Answer from the drawing. Dimensions are ordinates in mm from the lowest x, y and z of the part. Coordinates: 2 decimals unless noted, no trailing zeros. Order: outer loops, then holes, each group sorted by start corner. A loop starts at its lowest first (then second) coordinate and runs counter-clockwise, first axis right, second up. Notation, with made-up numbers: (-7.5, -28) - (12.5, -28) arc R36 cw to (12.5, 6) - close; hole circle Ø8 at (-8, 65.25). An arc over 180 degrees is marked (long way). Use a Markdown table: item, result. Add a question column.
Item 1: The mould has two halves that part along X. Classify the marked faces 1, 2, 3 and 4: released by +X, released by -X, zero draft, split by the parting line, or undercut.
Item 2: The part is cut by section B-B, the plane y = 1.3. Give the vertices of the cut face in (x, z).
Item 3: Flat-ended cylindrical pins translate along their axes: P1, Ø1, axis at x = 3.5, z = 4, coming from the -Y side; P2, Ø3, axis at x = 7, z = 6, coming from the -Y side. Find the tip coordinate at first contact, or state that the pin passes through.
Item 4: Find the intervals of material crossed by line 1 along X through (y, z) = (2.8, 5); line 2 along Z through (x, y) = (5, 2.15) (1 decimal); line 3 along X through (y, z) = (1.8, 4.25) (1 decimal), in increasing order.
Item 5: The part is cut by section A-A, the plane z = 5. Give the vertices of the cut face in (x, y), then the cut area to 3 significant figures.
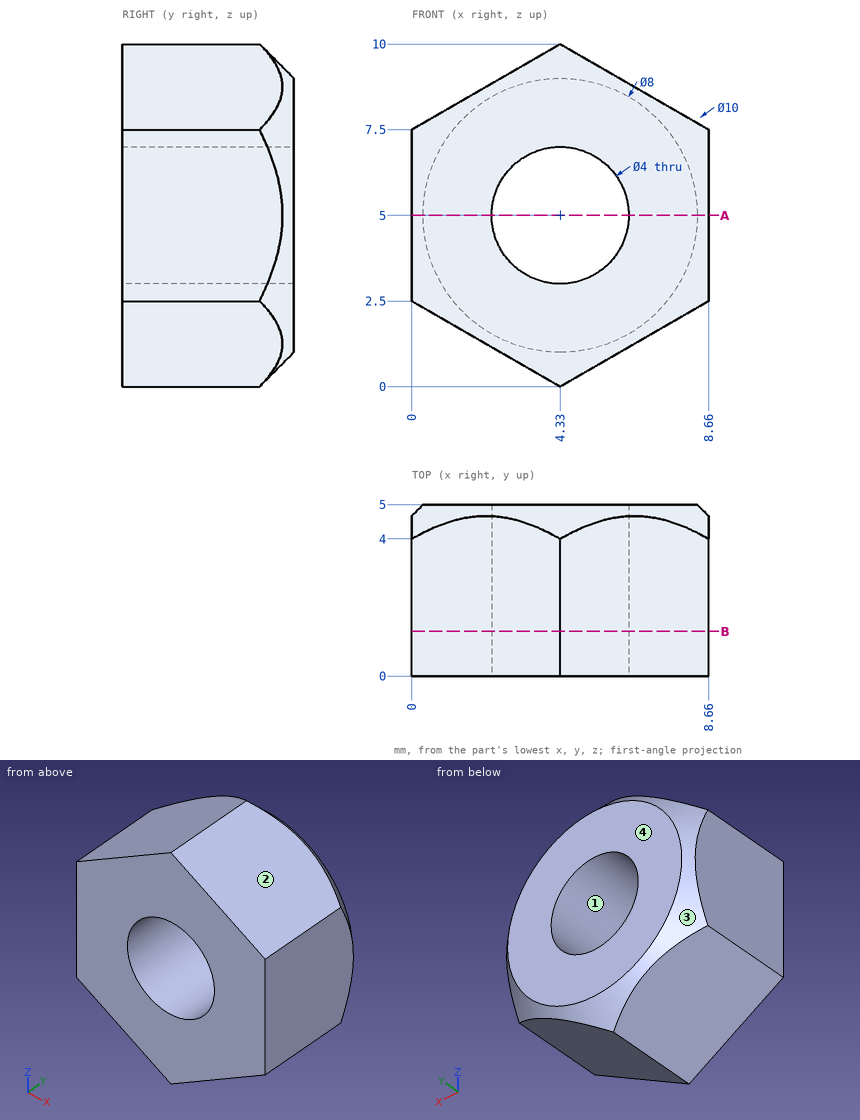
Solution:
| question | item | result |
|---|---|---|
| 1 | face 1 | undercut |
| 1 | face 2 | released by +X |
| 1 | face 3 | split by the parting line |
| 1 | face 4 | zero draft |
| 2 | outline | (0, 2.5) - (4.33, 0) - (8.66, 2.5) - (8.66, 7.5) - (4.33, 10) - (0, 7.5) - close; hole circle Ø4 at (4.33, 5) |
| 3 | P1 | passes through |
| 3 | P2 | stops at y = 0 |
| 4 | line 1 | x = 0 to 2.33, 6.33 to 8.66 |
| 4 | line 2 | z = 0.4 to 3.1, 6.9 to 9.6 |
| 4 | line 3 | x = 0 to 2.5, 6.2 to 8.7 |
| 5 | outline | (0, 0) - (2.33, 0) - (2.33, 5) - (0.33, 5) - (0, 4.67) - close; (6.33, 0) - (8.66, 0) - (8.66, 4.67) - (8.33, 5) - (6.33, 5) - close |
| 5 | area | 23.2 mm2 |
